For this review, take the finished solid that the model builds, in its own axes (mm). A direction names the side the tool comes from. Give positions to 0.01 mm unless a question says otherwise; leave off trailing zeros. Loops run counter-clockwise (first coordinate to the right, second up) from the corner with the lowest first, then second, coordinate; pieces in that order, holes last. Notation, with made-up numbers: (75.25, 44.5) - (127.25, 44.5) arc R16 cw to (127.25, 56.5) - close; hole circle Ø2 at (-11.75, -10.5). An arc over 180 degrees is marked (long way). Answer as CSV lines item,"result".
from build123d import *

# Parameters (mm, degrees)
F0_W        = 3.0256015398
F0_H        = 2.0134245381
F1_DEPTH    = 2
F0_W_2      = 3.0003240481
F0_H_2      = 2.0157374777
F0_H_3      = 2.019865565
F0_W_3      = 3.0242641605
F2_DEPTH    = 34
F3_DEPTH    = 34
F0_W_4      = 3.0575518031
F0_W_5      = 3.0562144239
F4_DEPTH    = 19
F5_T4_DEPTH = 178.7945589271
F5_T9_DEPTH = 178.7904308398
F7_F1_R     = 1.9999
F7_F2_R     = 1.9999
F7_F3_R     = 1.9999
F7_F4_R     = 1.9999
F7_F5_R     = 2
F7_F6_R     = 2
F7_F7_R     = 2
F8_F1_R     = 2


# Not quite as in the source:
# - a fillet or chamfer that OpenCascade refuses, or shapes differently, is made with other operations: its cross-section is extruded or revolved along the edge and cut away or added
# - two fillets or chamfers of one size are made in one step
# - a fillet or chamfer is up to 0.001 mm smaller than in the source, because OpenCascade refuses the exact size


with BuildPart() as f1:
    # F0 (on Top) → F1 (new body)
    with BuildSketch(Plane.XY):
        with Locations((-7.4871992301, 6.743287731)):
            Rectangle(F0_W, F0_H)
    extrude(amount=F1_DEPTH)



with BuildPart() as f1b:
    # F0 (on Top) → F1, piece 2 (new body)
    with BuildSketch(Plane.XY):
        with Locations((7.4998379759, 6.7421312612)):
            Rectangle(F0_W_2, F0_H_2)
    extrude(amount=F1_DEPTH)



with BuildPart() as f1c:
    # F0 (on Top) → F1, piece 3 (new body)
    with BuildSketch(Plane.XY):
        with Locations((7.4998379759, -6.7400672175)):
            Rectangle(F0_W_2, F0_H_3)
    extrude(amount=F1_DEPTH)


with BuildPart() as f1d:
    # F0 (on Top) → F1, piece 4 (new body)
    with BuildSketch(Plane.XY):
        with Locations((-7.4878679197, -6.7400672175)):
            Rectangle(F0_W_3, F0_H_3)
    extrude(amount=F1_DEPTH)


with BuildPart() as f2:
    # F0 (on Top) → F2 (new body)
    with BuildSketch(Plane.XY):
        Polygon((1.2222049991, -5.730134435), (1.2222049991, 5.7342625223), (1.2222049991, 7.5), (-1.2222049991, 7.5), (-1.2222049991, 5.7365754619), (-1.2222049991, -5.730134435), (-1.2222049991, -7.5), (1.2222049991, -7.5), align=None)
    extrude(amount=F2_DEPTH)


with BuildPart() as f1b_1:
    add(f1b.part)

    add(f1c.part)  # F3 merges F1c

    add(f2.part)  # F3 merges F2
    # F0 (on Top) → F3 (join)
    with BuildSketch(Plane.XY):
        Polygon((5.9996759519, 5.7342625223), (5.9996759519, 7.75), (-2.9181840364, 7.75), (-2.9181840364, 5.7365754619), (-1.2222049991, 5.7365754619), (-1.2222049991, 7.5), (1.2222049991, 7.5), (1.2222049991, 5.7342625223), align=None)
        Polygon((5.9996759519, -7.75), (5.9996759519, -5.730134435), (1.2222049991, -5.730134435), (1.2222049991, -7.5), (-1.2222049991, -7.5), (-1.2222049991, -5.730134435), (-2.9181840364, -5.730134435), (-2.9181840364, -7.75), align=None)
    extrude(amount=F3_DEPTH)


with BuildPart() as f1_1:
    add(f1.part)

    add(f1b_1.part)  # F4 merges F1b

    add(f1d.part)  # F4 merges F1d
    # F0 (on Top) → F4 (join)
    with BuildSketch(Plane.XY):
        with Locations((-4.4469599379, -6.7400672175)):
            Rectangle(F0_W_4, F0_H_3)
        with Locations((-4.4462912483, 6.743287731)):
            Rectangle(F0_W_5, F0_H)
    extrude(amount=F4_DEPTH)

    # F5: chamfer of 3 x 34 on 2 edges, made by hand


with BuildPart() as f5_tool2:
    # F5_s3 → F5_t4 (new body)
    with BuildSketch(Plane.XZ.offset(96.137346681)):
        Polygon((5.9996759519, 0), (2.9996759519, 34), (5.9996759519, 34), align=None)
    extrude(amount=-F5_T4_DEPTH)

    split(bisect_by=Plane.XY.offset(2), keep=Keep.TOP)


with BuildPart() as f1_2:
    add(f1_1.part)

    # F5_t1: cut F5_tool2
    add(f5_tool2.part, mode=Mode.SUBTRACT)


with BuildPart() as f5_tool7:
    # F5_s8 → F5_t9 (new body)
    with BuildSketch(Plane.XZ.offset(82.6530841587)):
        Polygon((5.9996759519, 0), (2.9996759519, 34), (5.9996759519, 34), align=None)
    extrude(amount=-F5_T9_DEPTH)

    split(bisect_by=Plane.XY.offset(2), keep=Keep.TOP)


with BuildPart() as f1_3:
    add(f1_2.part)

    # F5_t6: cut F5_tool7
    add(f5_tool7.part, mode=Mode.SUBTRACT)

    # F7: fillet of radius 2 on 8 edges, made by hand

    # F7_f1 (radius 2 in the source; OpenCascade refuses exactly that, so slightly less here)
    f7_f1_edges = [f1_3.edges().sort_by_distance(p)[0] for p in [
        (-9, -6.7400672175, 2),
    ]]
    fillet(f7_f1_edges, radius=F7_F1_R)

    # F7_f2 (radius 2 in the source; OpenCascade refuses exactly that, so slightly less here)
    f7_f2_edges = [f1_3.edges().sort_by_distance(p)[0] for p in [
        (9, -6.7400672175, 2),
    ]]
    fillet(f7_f2_edges, radius=F7_F2_R)

    # F7_f3 (radius 2 in the source; OpenCascade refuses exactly that, so slightly less here)
    f7_f3_edges = [f1_3.edges().sort_by_distance(p)[0] for p in [
        (9, 6.7421312612, 2),
    ]]
    fillet(f7_f3_edges, radius=F7_F3_R)

    # F7_f4 (radius 2 in the source; OpenCascade refuses exactly that, so slightly less here)
    f7_f4_edges = [f1_3.edges().sort_by_distance(p)[0] for p in [
        (-9, 6.743287731, 2),
    ]]
    fillet(f7_f4_edges, radius=F7_F4_R)

    # F7_f5
    f7_f5_edges = [f1_3.edges().sort_by_distance(p)[0] for p in [
        (-5.9743984602, 6.743287731, 19),
    ]]
    fillet(f7_f5_edges, radius=F7_F5_R)

    # F7_f6
    f7_f6_edges = [f1_3.edges().sort_by_distance(p)[0] for p in [
        (-2.9181840364, 6.743287731, 34),
    ]]
    fillet(f7_f6_edges, radius=F7_F6_R)

    # F7_f7
    f7_f7_edges = [f1_3.edges().sort_by_distance(p)[0] for p in [
        (-5.9757358395, -6.7400672175, 19),
    ]]
    fillet(f7_f7_edges, radius=F7_F7_R)

    # F8: fillet of radius 2 on 2 edges, made by hand

    # F8_f1
    f8_f1_edges = [f1_3.edges().sort_by_distance(p)[0] for p in [
        (2.9996759519, -6.7400672175, 34),
    ]]
    fillet(f8_f1_edges, radius=F8_F1_R)


solid = f1_3.part
1) Draft analysis for pull direction Y (two halves, no side actions). For faces 1 (the flat face through (6, 7, 2)), 2 (the flat face through (3, 5.734, 13)), 3 (the flat face through (0, -7.75, 13)), 4 (the flat face through (-3, -5.73, 13)), state which applies: pulls with the +Y half, pulls with the -Y half, needs draft (parallel to the pull), parting line crosses it, or undercut.
From the geometry:
face 1,"needs draft"
face 2,"undercut"
face 3,"pulls with the -Y half"
face 4,"undercut"
2) Consider section D-D on x = -4.5. Write out the cut boundary in (y, z).
From the geometry:
outline,"(-7.75, 0) - (-5.73, 0) - (-5.73, 18.93) - (-7.75, 18.93) - close; (5.74, 0) - (7.75, 0) - (7.75, 18.93) - (5.74, 18.93) - close"
3) Machinability: for faces 5 (the flat face through (-3, 5.737, 13)), 6 (the flat face through (3, -5.73, 13)), 7 (the flat face through (0, 1, 0)), 8 (the flat face through (-6.5, 6.8, 2)), which of the approach directions +Z, -Z, +X, -X, +Y, -Y give a long, thin tool a straight path to every point of the face, cutting with its end or side? Answer none if there is none.
From the geometry:
face 5,"+Z, -Z, -X"
face 6,"+Z, -Z, +X"
face 7,"-Z, +X, -X, +Y, -Y"
face 8,"+Z, -X, +Y, -Y"
4) Consider section C-C on z = 24. Write out the cut boundary in (x, y).
From the geometry:
outline,"(-2.92, -7.75) - (3.88, -7.75) - (3.88, -5.73) - (1.22, -5.73) - (1.22, 5.73) - (3.88, 5.73) - (3.88, 7.75) - (-2.92, 7.75) - (-2.92, 5.74) - (-1.22, 5.74) - (-1.22, -5.73) - (-2.92, -5.73) - close"
5) Insertion check: P1, Ø1.6, axis at y = 6.5, z = 25.5, coming from the -X side; P2, Ø0.5, axis at x = -6.5, y = -6.5, coming from the +Z side; P3, Ø1.5, axis at y = 3.5, z = 19.5, coming from the -X side; P4, Ø1, axis at x = 6.5, z = 10, coming from the -Y side. Each pin has a flat end and moves straight along its axis. Give the tip position at first contact, or say it passes through.
From the geometry:
P1,"stops at x = -2.92"
P2,"stops at z = 2"
P3,"stops at x = -1.22"
P4,"passes through"
6) Consider section A-A on x = 7.5. Write out the cut boundary in (y, z).
From the geometry:
outline,"(-7.75, 0) - (-5.73, 0) - (-5.73, 1.94) - (-7.75, 1.94) - close; (5.73, 0) - (7.75, 0) - (7.75, 1.94) - (5.73, 1.94) - close"
7) Wall thickness on line 1 (Y direction, x = 2.75, z = 31); line 2 (X direction, y = -4.75, z = 33.5); line 3 (Z direction, x = 6, y = -7): over which ranges is each line inside the solid? List them lowest first. Write a range as from..to.
From the geometry:
line 1,"y = -7.75..-5.73, 5.73..7.75"
line 2,"x = -1.22..1.22"
line 3,"z = 0..2"
